Model file for the job. Use its own axes, mm. A direction names the side the tool comes from. Round coordinates to 2 decimals unless told otherwise and drop trailing zeros. Loops run counter-clockwise (first coordinate to the right, second up) from the corner with the lowest first, then second, coordinate; pieces in that order, holes last. Notation, with made-up numbers: M 77.25,33.5 L 103.25,33.5 A28 ccw 103.25,72.5 Z; hole C -30,15.25 d6. An arc over 180 degrees is marked long. Answer in a Markdown table with one row per item.
from build123d import *

# Parameters (mm, degrees)
EXTRUDE_1_DEPTH     = 10
CUT_EXTRUDE_4_DEPTH = 85
SKETCH_6_R          = 1.5
CUT_EXTRUDE_5_DEPTH = 12.107026924
SKETCH_7_R          = 3.25
CUT_EXTRUDE_6_DEPTH = 8.107026924
SKETCH_8_R          = 8
EXTRUDE_2_DEPTH     = 30
SKETCH_9_R          = 3.5
CUT_EXTRUDE_7_DEPTH = 30
SKETCH_10_R         = 5.25
CUT_EXTRUDE_8_DEPTH = 24


with BuildPart() as part:
    # 草图1 → 凸台-拉伸1 (new body)
    with BuildSketch(Plane(origin=(0, 0, 0), x_dir=(1, 0, 0), z_dir=(0, 1, 0))):
        Polygon((-42, 5.5), (-42, 10.5), (42, 10.5), (42, 5.5), (42, -5.5), (31, -5.5), (31, 5.5), (-31, 5.5), (-31, -5.5), (-42, -5.5), align=None)
    extrude(amount=EXTRUDE_1_DEPTH)

    # 草图5 → 切除-拉伸4 (cut, through all)
    with BuildSketch(Plane.ZY.offset(42)):
        Polygon((-5.5, 10), (5.5, 5.996327423), (5.5, 10), align=None)
    extrude(amount=-CUT_EXTRUDE_4_DEPTH, mode=Mode.SUBTRACT)

    # 草图6 → 切除-拉伸5 (cut, through all)
    with BuildSketch(Plane(origin=(0, 13.15030494, -14.155391688), x_dir=(1, 0, 0), z_dir=(0, -0.939692621, -0.342020143))):
        with Locations((-36.5, 15.063853195)):
            Circle(SKETCH_6_R)
        with Locations((36.5, 15.063853195)):
            Circle(SKETCH_6_R)
    extrude(amount=CUT_EXTRUDE_5_DEPTH, mode=Mode.SUBTRACT)

    # 草图7 → 切除-拉伸6 (cut, through all)
    with BuildSketch(Plane(origin=(0, 3.303785806, 1.202479694), x_dir=(1, 0, 0), z_dir=(0, 0.939692621, 0.342020143))):
        with Locations((-36.5, 2.735533099)):
            Circle(SKETCH_7_R)
        with Locations((36.5, 2.735533099)):
            Circle(SKETCH_7_R)
    extrude(amount=-CUT_EXTRUDE_6_DEPTH, mode=Mode.SUBTRACT)

    # 草图8 → 凸台-拉伸2 (add)
    with BuildSketch(Plane.XZ):
        with Locations((0, -13.5)):
            Circle(SKETCH_8_R)
    extrude(amount=-EXTRUDE_2_DEPTH)

    # 草图9 → 切除-拉伸7 (cut)
    with BuildSketch(Plane(origin=(0, 30, 0), x_dir=(1, 0, 0), z_dir=(0, 1, 0))):
        with Locations((0, 13.5)):
            Circle(SKETCH_9_R)
    extrude(amount=-CUT_EXTRUDE_7_DEPTH, mode=Mode.SUBTRACT)

    # 草图10 → 切除-拉伸8 (cut)
    with BuildSketch(Plane.XZ):
        with Locations((0, -13.5)):
            Circle(SKETCH_10_R)
    extrude(amount=-CUT_EXTRUDE_8_DEPTH, mode=Mode.SUBTRACT)


solid = part.part
1. Mould opens along Z. For faces 3 (the cylindrical face through (35.3, 6.5, -1.5)), 4 (the flat face through (-3, 0, -7)), 5 (the flat face through (37, 3, 5.5)) say: +Z half, -Z half, draft (parallel to the pull), parting line (faces both ways), or undercut.
Verdict:
| item | result |
|---|---|
| face 3 | undercut |
| face 4 | draft |
| face 5 | +Z half |
2. Tool access for faces 1 (the cylindrical face through (-1.73, 14.79, -21.31)), 2 (the flat face through (-4, 24, -13)): list every direction of +Z, -Z, +X, -X, +Y, -Y with a clear straight run to the whole face (end or side of a thin tool).
Verdict:
| item | result |
|---|---|
| face 1 | +Y |
| face 2 | -Y |
3. Saw through at A-A (y = 25.5). Write the cut outline in (x, z).
Verdict:
| item | result |
|---|---|
| outline | C 0,-13.5 d16; hole C 0,-13.5 d7 |
4. Saw through at C-C (x = 23). Write the cut outline in (y, z).
Verdict:
| item | result |
|---|---|
| outline | M 0,-10.5 L 10,-10.5 L 10,-5.5 L 0,-5.5 Z |
5. Pin check, flat tips, straight feed: pin 1 (5 mm diameter, centred on x = -1, y = 5.5, fed in from +Z); pin 2 (3 mm diameter, centred on x = -25.5, y = 10, fed in from -Z); pin 3 (5 mm diameter, centred on y = 13.5, z = -17.5, fed in from +X). Stop position of each tip, or through.
Verdict:
| item | result |
|---|---|
| pin 1 | stops at z = -5.5 |
| pin 2 | stops at z = -10.5 |
| pin 3 | stops at x = 7.86 |
6. Wall check: probe 1 along Z at (x, y) = (0, 16); probe 2 along X at (y, z) = (28.35, -13.5); probe 3 along X at (y, z) = (6.5, 3.5). Give the ranges that are in metal, low to high.
Verdict:
| item | result |
|---|---|
| probe 1 | z = -21.5 to -18.75, -8.25 to -5.5 |
| probe 2 | x = -8 to -3.5, 3.5 to 8 |
| probe 3 | x = -42 to -31, 31 to 42 |
7. Saw through at B-B (z = -16). Write the cut outline in (x, y), and give its area (3 significant figures).
Verdict:
| item | result |
|---|---|
| outline | M -7.6,0 L -4.62,0 L -4.62,24 L -2.45,24 L -2.45,30 L -7.6,30 Z; M 2.45,24 L 4.62,24 L 4.62,0 L 7.6,0 L 7.6,30 L 2.45,30 Z |
| area | 205 mm² |
8. Saw through at D-D (y = 11.75). Write the cut outline in (x, z), and give its area (3 significant figures).
Verdict:
| item | result |
|---|---|
| outline | C 0,-13.5 d16; hole C 0,-13.5 d10.5 |
| area | 114 mm² |
